```python
from build123d import *

# Parameters (mm, degrees)
CROQUIS1_W              = 100
CROQUIS1_H              = 127.304752994
SALIENTE_EXTRUIR1_DEPTH = 3
CROQUIS2_W              = 4
CROQUIS2_H              = 34.992450208
SALIENTE_EXTRUIR2_DEPTH = 60
CROQUIS4_W              = 34.992450208
CROQUIS4_H              = 4
SALIENTE_EXTRUIR3_DEPTH = 40
CHAFL_N1_SIZE           = 10
REDONDEO1_R             = 2
CROQUIS5_R              = 5.3
CROQUIS5_R_2            = 1.8
CORTAR_EXTRUIR2_DEPTH   = 40


with BuildPart() as part:
    # Croquis1 → Saliente-Extruir1 (new body)
    with BuildSketch(Plane(origin=(0, 0, 0), x_dir=(1, 0, 0), z_dir=(0, 1, 0))):
        Rectangle(CROQUIS1_W, CROQUIS1_H)
    extrude(amount=SALIENTE_EXTRUIR1_DEPTH)

    # Croquis2 → Saliente-Extruir2 (add)
    with BuildSketch(Plane.XZ):
        with Locations((33.610839978, 0)):
            Rectangle(CROQUIS2_W, CROQUIS2_H)
    extrude(amount=SALIENTE_EXTRUIR2_DEPTH)

    # Croquis4 → Saliente-Extruir3 (add)
    with BuildSketch(Plane(origin=(35.610839978, 0, 0), x_dir=(0, 0, -1), z_dir=(1, 0, 0))):
        with Locations((0, -58)):
            Rectangle(CROQUIS4_W, CROQUIS4_H)
    extrude(amount=SALIENTE_EXTRUIR3_DEPTH)

    # Chaflán1
    chafl_n1_edges = [part.edges().sort_by_distance(p)[0] for p in [
        (31.610839978, 0, 0),
    ]]
    chamfer(chafl_n1_edges, length=CHAFL_N1_SIZE)

    # Redondeo1
    redondeo1_edges = [part.edges().sort_by_distance(p)[0] for p in [
        (31.610839978, -60, 0),
        (35.610839978, -56, 0),
    ]]
    fillet(redondeo1_edges, radius=REDONDEO1_R)

    # Croquis5 → Cortar-Extruir2 (cut)
    with BuildSketch(Plane.XZ.offset(60)):
        with Locations((60.298029847, 0)):
            Circle(CROQUIS5_R)
        with Locations((67.72265105, -7.424621202)):
            Circle(CROQUIS5_R_2)
        with Locations((52.873408645, -7.424621202)):
            Circle(CROQUIS5_R_2)
        with Locations((52.873408645, 7.424621202)):
            Circle(CROQUIS5_R_2)
        with Locations((67.72265105, 7.424621202)):
            Circle(CROQUIS5_R_2)
    extrude(amount=-CORTAR_EXTRUIR2_DEPTH, mode=Mode.SUBTRACT)


solid = part.part
```
For this review, take the finished solid that the model builds, in its own axes (mm). A direction names the side the tool comes from. Round coordinates to 2 decimals unless told otherwise and drop trailing zeros. Order: outer loops, then holes, each group sorted by start corner. A loop starts at its lowest first (then second) coordinate and runs counter-clockwise, first axis right, second up.
Q1. We need section A-A, the plane z = 0. Give the boundary of the cut face in (x, y), plus the area to 3 significant figures.
Findings below:
outline: (-50, 0) - (21.61, 0) - (31.61, -10) - (31.61, -58) arc R2 ccw to (33.61, -60) - (55, -60) - (55, -56) - (37.61, -56) arc R2 cw to (35.61, -54) - (35.61, 0) - (50, 0) - (50, 3) - (-50, 3) - close; (65.6, -60) - (75.61, -60) - (75.61, -56) - (65.6, -56) - close
area: 708 mm2
Q2. Mouldability with a two-part tool opening along Z and no side actions: class faces 4 (the flat face through (-50, 1, 1)), 5 (the cylindrical face through (54.536, -58.028, -8.114)), 6 (the flat face through (34, -37, -17.496)) as pulls with the +Z half, pulls with the -Z half, needs draft (parallel to the pull), parting line crosses it, or undercut.
Findings below:
face 4: needs draft
face 5: undercut
face 6: pulls with the -Z half
Q3. We need section C-C, the plane y = -44.5. Give the boundary of the cut face in (x, z).
Findings below:
outline: (31.61, -17.5) - (35.61, -17.5) - (35.61, 17.5) - (31.61, 17.5) - close
Q4. Machinability: for faces 1 (the flat face through (34, -37, 17.496)), 2 (the flat face through (50, 1, 1)), 3 (the flat face through (35.611, -27, 0)), which of the approach directions +Z, -Z, +X, -X, +Y, -Y give a long, thin tool a straight path to every point of the face, cutting with its end or side? Answer none if there is none.
Findings below:
face 1: +Z, +X, -X, -Y
face 2: +Z, -Z, +X, +Y
face 3: +Z, -Z, +X
Q5. Insertion check: P1, Ø10.5, axis at x = 65.5, z = -6.5, coming from the +Y side; P2, Ø2.5, axis at y = 1, z = -12.5, coming from the +X side; P3, Ø6.5, axis at x = 60.3, z = 0, coming from the +Y side; P4, Ø10.5, axis at y = -17, z = -5.5, coming from the +X side. Each pin has a flat end and moves straight along its axis. Give the tip position at first contact, or say it passes through.
Findings below:
P1: stops at y = -56
P2: stops at x = 50
P3: passes through
P4: stops at x = 35.61
Q6. Wall thickness on line 1 (Y direction, x = -10, z = 7); line 2 (Y direction, x = 41, z = 12.5); line 3 (Z direction, x = 34.5, y = -15): over which ranges is each line inside the solid? List them lowest first.
Findings below:
line 1: y = 0 to 3
line 2: y = -60 to -56, 0 to 3
line 3: z = -17.5 to 17.5
Q7. We need section B-B, the plane x = -19. Give the boundary of the cut face in (y, z).
Findings below:
outline: (0, -63.65) - (3, -63.65) - (3, 63.65) - (0, 63.65) - close
